Check sheet for the modelled part. Datum: model origin and axes. Units: mm. Round coordinates to 2 decimals unless told otherwise and drop trailing zeros. Loops run counter-clockwise (first coordinate to the right, second up) from the corner with the lowest first, then second, coordinate; pieces in that order, holes last. Notation, with made-up numbers: (79.25, 64.5) - (104.25, 64.5) arc R15 cw to (104.25, 72.5) - close; hole circle Ø9 at (37.5, 36.25). An arc over 180 degrees is marked (long way). Answer in a Markdown table with one row per item. Add a question column.
(1) Cross-section at A-A on z = -49.5. Enter the section's corners in (x, y).
(2) Thickness scan on line 1 along X through (y, z) = (12.5, 75); line 2 along X through (y, z) = (5, -57); line 3 along Z through (x, y) = (-25, 14.25). Record the ranges inside material, lowest first.
(3) Cross-section at C-C on z = 125. Enter the section's corners in (x, y), then the cut area to 3 significant figures.
(4) Gauge pin test, flat ends, axial feed: pin 1 (13 mm diameter, centred on x = -125, z = -75, fed in from -Y); pin 2 (6 mm diameter, centred on x = -125, z = -125, fed in from -Y). Record the tip position at first contact, or that the pin passes through.
(5) Cross-section at D-D on x = 125. Enter the section's corners in (y, z).
(6) Cross-section at B-B on x = 25. Enter the section's corners in (y, z), then the cut area to 4 significant figures.
Autodesk Inventor part; units mm, degrees
ref_plane "YZ Plane" through (0, 0, 0) normal (1, 0, 0) x (0, 1, 0)
ref_plane "XZ Plane" through (0, 0, 0) normal (0, 1, 0) x (-1, 0, 0)
ref_plane "XY Plane" through (0, 0, 0) normal (0, 0, 1) x (1, 0, 0)
sketch "Sketch1" plane through (0, 0, 0) normal (0, 1, 0) x (-1, 0, 0)
  line L0 (130, 135) -> (-130, 135)
  line L1 (-135, 130) -> (-135, -130)
  line L2 (-130, -135) -> (130, -135)
  line L3 (135, -130) -> (135, 130)
  line L4 (135, 135) -> (-135, -135) construction
  line L5 (-135, 135) -> (135, -135) construction
  arc A0 (135, 130) -> (130, 135) centre (130, 130) ccw
  arc A1 (130, -135) -> (135, -130) centre (130, -130) ccw
  arc A2 (-135, -130) -> (-130, -135) centre (-130, -130) ccw
  arc A3 (-130, 135) -> (-135, 130) centre (-130, 130) ccw
  point P0 (0, 0)
  point P1 (0, 0)
  dimension "d0" = 270
  dimension "d1" = 270
  dimension "d2" = 5
  dimension "d3" = 5
  dimension "d4" = 5
  dimension "d5" = 5
extrude "Extrusion1" add sketch "Sketch1" along normal blind 20
sketch "Sketch2" plane through (0, 20, 0) normal (0, 1, 0) x (1, 0, 0)
  line L0 (-37.5, -62.5) -> (37.5, -62.5)
  line L1 (37.5, -62.5) -> (37.5, 62.5)
  line L2 (37.5, 62.5) -> (-37.5, 62.5)
  line L3 (-37.5, 62.5) -> (-37.5, -62.5)
  line L4 (-37.5, -62.5) -> (37.5, 62.5) construction
  line L5 (37.5, -62.5) -> (-37.5, 62.5) construction
  point P0 (0, 0)
  dimension "d8" = 75
  dimension "d9" = 125
extrude "Extrusion2" cut sketch "Sketch2" against normal blind 65.25
sketch "Sketch3" plane through (0, 20, 0) normal (0, 1, 0) x (1, 0, 0)
  line L0 (-50.5, -77.5) -> (50.5, -77.5)
  line L1 (52.5, -75.5) -> (52.5, 75.5)
  line L2 (50.5, 77.5) -> (-50.5, 77.5)
  line L3 (-52.5, 75.5) -> (-52.5, -75.5)
  line L4 (-52.5, -77.5) -> (52.5, 77.5) construction
  line L5 (52.5, -77.5) -> (-52.5, 77.5) construction
  arc A0 (-50.5, 77.5) -> (-52.5, 75.5) centre (-50.5, 75.5) ccw
  arc A1 (52.5, 75.5) -> (50.5, 77.5) centre (50.5, 75.5) ccw
  arc A2 (50.5, -77.5) -> (52.5, -75.5) centre (50.5, -75.5) ccw
  arc A3 (-52.5, -75.5) -> (-50.5, -77.5) centre (-50.5, -75.5) ccw
  point P0 (0, 0)
  dimension "d12" = 105
  dimension "d13" = 155
  dimension "d14" = 2
extrude "Extrusion3" cut sketch "Sketch3" against normal blind 2.5
sketch "Sketch5" plane through (0, 20, 0) normal (0, 1, 0) x (1, 0, 0)
  circle A0 centre (-70, 65) radius 5
  circle A1 centre (70, 65) radius 5
  circle A2 centre (70, -65) radius 5
  circle A3 centre (-70, -65) radius 5
  point P0 (0, 0)
  dimension "d17" = 10
  dimension "d18" = 10
  dimension "d19" = 10
  dimension "d20" = 10
hole "Hole1" at (-70, 20, 65) at (-70, 20, -65) at (70, 20, -65) at (70, 20, 65) direction (0, -1, 0) diameter 10 end through all
sketch "Sketch6" plane through (0, 20, 0) normal (0, 1, 0) x (1, 0, 0)
  point P0 (0, 0)
sketch "Sketch7" plane through (0, 20, 0) normal (0, 1, 0) x (1, 0, 0)
  line L0 (-135, 130) -> (-135, -130)
  line L1 (130, 135) -> (-130, 135)
  line L2 (135, -130) -> (135, 130)
  circle A0 centre (70, -65) radius 5
  circle A1 centre (70, 65) radius 5
  circle A2 centre (-70, 65) radius 5
  circle A3 centre (-70, -65) radius 5
  line L3 (52.5, 75.5) -> (52.5, -75.5)
  arc A4 (50.5, -77.5) -> (52.5, -75.5) centre (50.5, -75.5) ccw
  line L4 (50.5, -77.5) -> (-50.5, -77.5)
  arc A5 (-52.5, -75.5) -> (-50.5, -77.5) centre (-50.5, -75.5) ccw
  line L5 (-52.5, -75.5) -> (-52.5, 75.5)
  arc A6 (-50.5, 77.5) -> (-52.5, 75.5) centre (-50.5, 75.5) ccw
  line L6 (-50.5, 77.5) -> (50.5, 77.5)
  arc A7 (52.5, 75.5) -> (50.5, 77.5) centre (50.5, 75.5) ccw
  arc A8 (130, -135) -> (135, -130) centre (130, -130) ccw
  line L7 (135, -130) -> (135, 130)
  arc A9 (135, 130) -> (130, 135) centre (130, 130) ccw
  line L8 (130, 135) -> (-130, 135)
  arc A10 (-130, 135) -> (-135, 130) centre (-130, 130) ccw
  line L9 (-135, 130) -> (-135, -130)
  arc A11 (-135, -130) -> (-130, -135) centre (-130, -130) ccw
  line L10 (-130, -135) -> (130, -135)
  circle A12 centre (-125, -125) radius 5
  circle A13 centre (-125, -75) radius 5
  circle A14 centre (-125, -25) radius 5
  circle A15 centre (-125, 25) radius 5
  circle A16 centre (-125, 75) radius 5
  circle A17 centre (-125, 125) radius 5
  circle A18 centre (125, 75) radius 5
  circle A19 centre (125, 25) radius 5
  circle A20 centre (125, -25) radius 5
  circle A21 centre (125, -75) radius 5
  circle A22 centre (125, -125) radius 5
  circle A23 centre (-75, 125) radius 5
  circle A24 centre (75, 125) radius 5
  circle A25 centre (-75, -125) radius 5
  circle A26 centre (75, -125) radius 5
  circle A27 centre (125, 125) radius 5
  circle A28 centre (-25, 125) radius 5
  circle A29 centre (25, 125) radius 5
  circle A30 centre (-25, -125) radius 5
  circle A31 centre (25, -125) radius 5
  point P0 (0, 0)
  point P1 (0, 135)
  point P2 (0, 135)
  dimension "d34" = 10
  dimension "d36" = 10
  dimension "d37" = 10
  dimension "d39" = 10
  dimension "d40" = 10
  dimension "d49" = 50
  dimension "d50" = 50
  dimension "d52" = 50
  dimension "d53" = 50
  dimension "d54" = 10
  dimension "d55" = 10
  dimension "d56" = 10
  dimension "d57" = 10
  dimension "d58" = 10
  dimension "d59" = 50
  dimension "d60" = 10
  dimension "d63" = 10
  dimension "d64" = 10
  dimension "d65" = 10
  dimension "d66" = 10
  dimension "d67" = 10
  dimension "d68" = 10
  dimension "d69" = 10
  dimension "d70" = 10
  dimension "d72" = 10
  dimension "d73" = 10
  dimension "d74" = 10
  dimension "d75" = 50
  dimension "d76" = 10
  dimension "d77" = 50
  dimension "d78" = 10
  dimension "d79" = 50
  dimension "d80" = 10
  dimension "d81" = 10
  dimension "d82" = 10
  dimension "d83" = 50
  dimension "d84" = 50
  dimension "d85" = 10
  dimension "d86" = 50
  dimension "d87" = 75
  dimension "d88" = 50
  dimension "d89" = 10
  dimension "d90" = 75
  dimension "d91" = 10
  dimension "d92" = 50
  dimension "d93" = 50
  dimension "d94" = 10
  dimension "d95" = 10
  dimension "d96" = 10
  dimension "d97" = 10
  dimension "d98" = 10
  dimension "d99" = 50
  dimension "d100" = 50
  dimension "d101" = 50
  dimension "d102" = 10
  dimension "d103" = 10
  dimension "d104" = 10
  dimension "d105" = 10
  dimension "d106" = 50
  dimension "d107" = 50
  dimension "d108" = 50
hole "Hole2" at (-125, 20, -125) at (-75, 20, -125) at (-25, 20, -125) at (25, 20, -125) at (75, 20, -125) at (125, 20, -125) at (125, 20, -75) at (125, 20, -25) at (125, 20, 25) at (125, 20, 75) at (125, 20, 125) at (75, 20, 125) at (25, 20, 125) at (-25, 20, 125) at (-75, 20, 125) at (-125, 20, 125) at (-125, 20, -75) at (-125, 20, -25) at (-125, 20, 25) at (-125, 20, 75) direction (0, -1, 0) diameter 10 end through all
sketch "Sketch8" plane through (0, 20, 0) normal (0, 1, 0) x (1, 0, 0)
  point P0 (0, 0)
thread "Thread1"
thread "Thread2"
thread "Thread3"
thread "Thread4"
properties part number "Impact Test Fixturev4 BS EN 6038 assemblyFEA" material "Steel, Carbon"
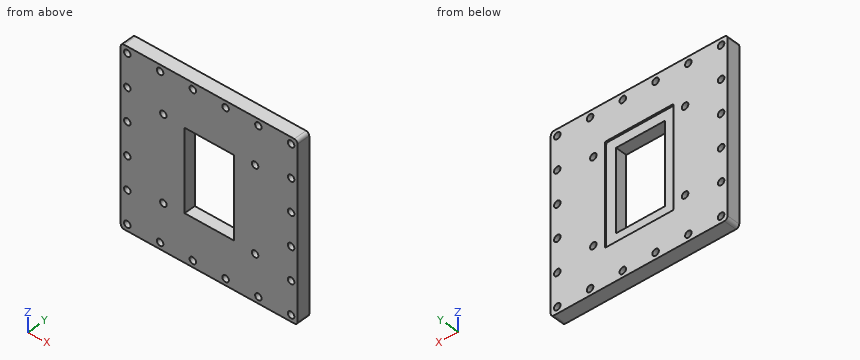
Answers:
| question | item | result |
|---|---|---|
| 1 | outline | (-135, 0) - (-37.5, 0) - (-37.5, 17.5) - (-52.5, 17.5) - (-52.5, 20) - (-135, 20) - close; (37.5, 0) - (135, 0) - (135, 20) - (52.5, 20) - (52.5, 17.5) - (37.5, 17.5) - close |
| 2 | line 1 | x = -135 to -130, -120 to 120, 130 to 135 |
| 2 | line 2 | x = -135 to -37.5, 37.5 to 135 |
| 2 | line 3 | z = -135 to -130, -120 to -62.5, 62.5 to 120, 130 to 135 |
| 3 | outline | (-135, 0) - (-130, 0) - (-130, 20) - (-135, 20) - close; (-120, 0) - (-80, 0) - (-80, 20) - (-120, 20) - close; (-70, 0) - (-30, 0) - (-30, 20) - (-70, 20) - close; (-20, 0) - (20, 0) - (20, 20) - (-20, 20) - close; (30, 0) - (70, 0) - (70, 20) - (30, 20) - close; (80, 0) - (120, 0) - (120, 20) - (80, 20) - close; (130, 0) - (135, 0) - (135, 20) - (130, 20) - close |
| 3 | area | 4,200 mm^2 |
| 4 | pin 1 | stops at y = 0 |
| 4 | pin 2 | passes through |
| 5 | outline | (0, -135) - (20, -135) - (20, -130) - (0, -130) - close; (0, -120) - (20, -120) - (20, -80) - (0, -80) - close; (0, -70) - (20, -70) - (20, -30) - (0, -30) - close; (0, -20) - (20, -20) - (20, 20) - (0, 20) - close; (0, 30) - (20, 30) - (20, 70) - (0, 70) - close; (0, 80) - (20, 80) - (20, 120) - (0, 120) - close; (0, 130) - (20, 130) - (20, 135) - (0, 135) - close |
| 6 | outline | (0, -135) - (20, -135) - (20, -130) - (0, -130) - close; (0, -120) - (20, -120) - (20, -77.5) - (17.5, -77.5) - (17.5, -62.5) - (0, -62.5) - close; (0, 62.5) - (17.5, 62.5) - (17.5, 77.5) - (20, 77.5) - (20, 120) - (0, 120) - close; (0, 130) - (20, 130) - (20, 135) - (0, 135) - close |
| 6 | area | 2,425 mm^2 |
